from build123d import *

# Parameters (mm, degrees)
BODYSKE_R      = 1.5
BASEBODY_DEPTH = 3
FILLET1_R      = 3
FILLET2_R      = 2.1


with BuildPart() as part:
    # BodySke → BaseBody (new body)
    with BuildSketch(Plane.XY):
        with BuildLine():
            Line((-1.5, -47.226184474), (-1.5, -56.726184474))
            Line((-1.5, -56.726184474), (-7.5, -56.726184474))
            Line((-7.5, -56.726184474), (-7.5, -50.774419011))
            ThreePointArc((-7.5, -50.774419011), (0, 56.25), (7.5, -50.774419011))
            Line((7.5, -50.774419011), (7.5, -56.726184474))
            Line((7.5, -56.726184474), (1.5, -56.726184474))
            Line((1.5, -56.726184474), (1.5, -47.226184474))
            ThreePointArc((1.5, -47.226184474), (0, 47.25), (-1.5, -47.226184474))
        make_face()
        with Locations((-4.5, -53.750301743)):
            Circle(BODYSKE_R, mode=Mode.SUBTRACT)
        with Locations(Location((4.5, -53.750301743, 0), (0, 0, 180))):
            Circle(BODYSKE_R, mode=Mode.SUBTRACT)
    extrude(amount=BASEBODY_DEPTH)

    # Fillet1
    fillet1_edges = [part.edges().sort_by_distance(p)[0] for p in [
        (-7.5, -50.774419011, 1.5),
        (7.5, -50.774419011, 1.5),
    ]]
    fillet(fillet1_edges, radius=FILLET1_R)

    # Fillet2
    fillet2_edges = [part.edges().sort_by_distance(p)[0] for p in [
        (-7.5, -56.726184474, 1.5),
        (7.5, -56.726184474, 1.5),
    ]]
    fillet(fillet2_edges, radius=FILLET2_R)


solid = part.part
Geometry check sheet. Reference: the model listing, model coordinates, mm. A direction names the side the tool comes from. Round coordinates to 2 decimals unless told otherwise and drop trailing zeros. Loops run counter-clockwise (first coordinate to the right, second up) from the corner with the lowest first, then second, coordinate; pieces in that order, holes last. Notation, with made-up numbers: (22, -31) - (68, -31) arc R24 cw to (68, -6) - close; hole circle Ø7 at (-38, -14.75). An arc over 180 degrees is marked (long way). One line per question, with ' | ' between items. Start each with the question number.
1. Cross-section at D-D on x = 0. Record the cut outline in (y, z), then the cut area to 3 significant figures.
2. Cross-section at B-B on x = -32. Record the cut outline in (y, z).
3. Tool access check on faces 4 (the face through (-1.5, -52, 1)), 5 (the face through (4.695, -55.238, 1.479)). Record the directions out of +Z, -Z, +X, -X, +Y, -Y that give a thin tool (end or side, any length) a straight path to the whole face; none if there is none.
4. Cross-section at A-A on y = 40. Record the cut outline in (x, z).
5. Draft check along Y on faces 1 (the face through (-3, -56.726, 1)), 2 (the face through (1.5, -52, 1)), 3 (the face through (-4.825, -55.215, 1.479)). Enter one of: released by +Y, released by -Y, zero draft, split by the parting line, or undercut.
6. Depth check by flat-ended pin: pin 1 (1 mm diameter, centred on x = 30.5, z = 0.5, fed in from +Y); pin 2 (1.5 mm diameter, centred on x = -6.5, z = 0.5, fed in from -Y); pin 3 (1.5 mm diameter, centred on y = -44, z = 1.5, fed in from -X). Enter the tip coordinate at first touch or a pass-through.
7. Cross-section at C-C on z = 2.55. Record the cut outline in (x, y) (3 decimals), then the cut area to 3 significant figures.
8. Scan lines: line 1 (Y direction, x = 4.5, z = 2.15); line 2 (Y direction, x = 36, z = 0.5); line 3 (X direction, y = -11, z = 1.1). Record each from-to range of solid material in increasing order. Write a range as [from, to].
Taken from the geometry:
1) outline: (47.25, 0) - (56.25, 0) - (56.25, 3) - (47.25, 3) - close | area: 27.0 mm²
2) outline: (-40.74, 0) - (-34.76, 0) - (-34.76, 3) - (-40.74, 3) - close; (34.76, 0) - (45.69, 0) - (45.69, 3) - (34.76, 3) - close
3) face 4: +Z, -Z, -Y | face 5: +Z, -Z
4) outline: (-38.52, 0) - (-25.15, 0) - (-25.15, 3) - (-38.52, 3) - close; (25.15, 0) - (38.52, 0) - (38.52, 3) - (25.15, 3) - close
5) face 1: released by -Y | face 2: zero draft | face 3: undercut
6) pin 1: y = 47.1 | pin 2: y = -56.7 | pin 3: x = -28.3
7) outline: (-9.945, -50.372) arc R3 cw to (-7.5, -53.321) - (-7.5, -54.626) arc R2.1 ccw to (-5.4, -56.726) - (-1.5, -56.726) - (-1.5, -47.226) arc R47.25 cw (long way) to (1.5, -47.226) - (1.5, -56.726) - (5.4, -56.726) arc R2.1 ccw to (7.5, -54.626) - (7.5, -53.321) arc R3 cw to (9.945, -50.372) arc R53.775 ccw (long way) to start; hole circle Ø3 at (-4.5, -53.75); hole circle Ø3 at (4.5, -53.75) | area: 2,110 mm²
8) line 1: [-56.73, -55.25], [-52.25, -47.04], [47.04, 56.06] | line 2: [-37.47, -30.6], [30.6, 42.42] | line 3: [-52.06, -45.95], [45.95, 52.06]
